Work out the finished part from the listing and answer in its coordinate system (mm). A direction names the side the tool comes from. Coordinates: 2 decimals unless noted, no trailing zeros. Order: outer loops, then holes, each group sorted by start corner. A loop starts at its lowest first (then second) coordinate and runs counter-clockwise, first axis right, second up. Notation, with made-up numbers: M 68.25,1.25 L 108.25,1.25 A7 cw 108.25,12.25 Z; hole C 51,-6.75 d9. An arc over 180 degrees is marked long. Write item = value, one per line. Start each with the question number.
Q1. Determine the mould class of faces 1 (the flat face through (-24.193, -41.132, 2.465)), 2 (the flat face through (24.193, 41.132, 2.465)), 3 (the cylindrical face through (41.745, 23.601, -0.253)) for opening direction Y: released by +Y, released by -Y, zero draft, split by the parting line, or undercut.
Q2. A tool of negligible diameter and unlimited length cuts with its end or side. For faces 4 (the flat face through (46, -19, 2)), 5 (the flat face through (-22.656, -38.519, 2.465)), 6 (the flat face through (-23.52, 41.52, 2.46)), from which of +Z, -Z, +X, -X, +Y, -Y can it reach the whole face along a straight path? Write none if from no direction.
Q3. Each of these flat-tipped pins is pushed along its axis until it touches: P1, Ø6.5, axis at x = 39.84, y = -23, coming from the +Z side; P2, Ø4, axis at y = 21, z = 3, coming from the -X side; P3, Ø4, axis at y = 12, z = 1.5, coming from the -X side; P4, Ø3.5, axis at x = 46.5, z = 2.5, coming from the -Y side. Where does it stop, or does it pass through?
Q4. Straight lines are drawn through the part: line 1 along Z through (x, y) = (13, -14.5); line 2 along X through (y, z) = (-47, -1.25); line 3 along X through (y, z) = (-46, -0.4). For each, find the intervals that lie inside material, in ascending order.
Q5. Find section C-C on y = 16.5. Give the vertices of the cut face in (x, z), and give its area (3 significant figures).
Q6. Find section B-B on z = 2.5. Give the vertices of the cut face in (x, y), and give its area (3 significant figures).
Q7. Find section A-A on y = -23. Give the vertices of the cut face in (x, z).
Q8. Find section D-D on x = -29.5. Give the vertices of the cut face in (y, z).
```python
from build123d import *

# Parameters (mm, degrees)
CYLINDER050_R            = 2
CYLINDER050_DEPTH        = 21
ARRAY002_COUNT           = 6
CYLINDER043_R            = 1.2
CYLINDER043_DEPTH        = 10
PRISM002_DEPTH           = 3
PRISM002_PLACEMENT_ANGLE = 30
BOX010_W                 = 5
BOX010_H                 = 38
BOX010_DEPTH             = 10
PRISM004_DEPTH           = 11
PRISM004_PLACEMENT_ANGLE = 30
PRISM003_DEPTH           = 5
PRISM003_PLACEMENT_ANGLE = 30
CHAMFER007_SIZE          = 2.5


with BuildPart() as agujeros_tornillos_tapa_inferior:
    # Cylinder050 → Cylinder050 (new body)
    with BuildSketch(Plane(origin=(0, -46, -8), x_dir=(1, 0, 0), z_dir=(0, 0, 1))):
        Circle(CYLINDER050_R)
    extrude(amount=CYLINDER050_DEPTH)

    # Array002: agujeros tornillos tapa inferior ×6 about axis
    array002_axis = Axis((0, 0, 0), (0, 0, 1))


with BuildPart() as agujeros_tornillos_tapa_inferior_1:
    add(agujeros_tornillos_tapa_inferior.part)
    for i in range(1, ARRAY002_COUNT):
        add(agujeros_tornillos_tapa_inferior.part.rotate(array002_axis, i * 360 / ARRAY002_COUNT))


with BuildPart() as cilindro019:
    # Cylinder043 → Cylinder043 (new body)
    with BuildSketch(Plane.XY.offset(-6)):
        Circle(CYLINDER043_R)
    extrude(amount=CYLINDER043_DEPTH)


with BuildPart() as obj1:
    # Prism002 → Prism002 (new body)
    with BuildSketch(Plane.XY):
        Polygon((58.5, 0), (29.25, 50.662486), (-29.25, 50.662486), (-58.5, 0), (-29.25, -50.662486), (29.25, -50.662486), align=None)
    extrude(amount=PRISM002_DEPTH)


with BuildPart() as obj1_1:
    # Prism002 placement: moved
    add(obj1.part.moved(Location((0, 0, -3))).rotate(Axis((0, 0, -3), (0, 0, 1)), PRISM002_PLACEMENT_ANGLE))

    # Cut011: cut Cilindro019
    add(cilindro019.part, mode=Mode.SUBTRACT)


with BuildPart() as cubo007:
    # Box010 → Box010 (new body)
    with BuildSketch(Plane(origin=(43.7, -19, 0), x_dir=(1, 0, 0), z_dir=(0, 0, 1))):
        with Locations((2.5, 19)):
            Rectangle(BOX010_W, BOX010_H)
    extrude(amount=BOX010_DEPTH)


with BuildPart() as tapa002:
    # Prism004 → Prism004 (new body)
    with BuildSketch(Plane.XY):
        Polygon((51.6, 0), (25.8, 44.686911), (-25.8, 44.686911), (-51.6, 0), (-25.8, -44.686911), (25.8, -44.686911), align=None)
    extrude(amount=PRISM004_DEPTH)


with BuildPart() as tapa002_1:
    # Prism004 placement: moved
    add(tapa002.part.rotate(Axis((0, 0, 0), (0, 0, 1)), PRISM004_PLACEMENT_ANGLE))


with BuildPart() as obj2:
    # Prism003 → Prism003 (new body)
    with BuildSketch(Plane.XY):
        Polygon((55.1, 0), (27.55, 47.718), (-27.55, 47.718), (-55.1, 0), (-27.55, -47.718), (27.55, -47.718), align=None)
    extrude(amount=PRISM003_DEPTH)


with BuildPart() as obj2_1:
    # Prism003 placement: moved
    add(obj2.part.rotate(Axis((0, 0, 0), (0, 0, 1)), PRISM003_PLACEMENT_ANGLE))

    # Cut006: cut tapa002
    add(tapa002_1.part, mode=Mode.SUBTRACT)

    # Cut007: cut Cubo007
    add(cubo007.part, mode=Mode.SUBTRACT)

    # Fusion006: union obj1
    add(obj1_1.part)

    # Cut021: cut agujeros tornillos tapa inferior
    add(agujeros_tornillos_tapa_inferior_1.part, mode=Mode.SUBTRACT)

    # Chamfer007
    chamfer007_edges = [obj2_1.edges().sort_by_distance(p)[0] for p in [
        (-2, -46, -3),
        (38.837169, -24.732051, -3),
        (2, 46, -3),
        (-38.837169, 24.732051, -3),
        (-40.837169, -21.267949, -3),
        (40.837169, 21.267949, -3),
    ]]
    chamfer(chamfer007_edges, length=CHAMFER007_SIZE)


solid = obj2_1.part
```
Findings below:
q1.face_1 = released by -Y
q1.face_2 = released by +Y
q1.face_3 = undercut
q2.face_4 = +Z, +X
q2.face_5 = +Z
q2.face_6 = +Z, -X, +Y
q3.P1 = 0
q3.P2 = -47.72
q3.P3 = -50.66
q3.P4 = -29.26
q4.line_1 = -3 to 0
q4.line_2 = -19.92 to -2.56, 2.56 to 19.92
q4.line_3 = -21.65 to -2, 2 to 21.65
q5.outline = M -50.66,-3 L 50.66,-3 L 50.66,0 L -44.69,0 L -44.69,5 L -47.72,5 L -47.72,0 L -50.66,0 Z
q5.area = 319 mm^2
q6.outline = M -47.72,-27.55 L 0,-55.1 L 47.72,-27.55 L 47.72,-19 L 44.69,-19 L 44.69,-25.8 L 0,-51.6 L -44.69,-25.8 L -44.69,25.8 L 0,51.6 L 44.69,25.8 L 44.69,19 L 47.72,19 L 47.72,27.55 L 0,55.1 L -47.72,27.55 Z
q6.area = 855 mm^2
q7.outline = M -50.66,-3 L -44.34,-3 L -41.84,-0.5 L -41.84,0 L -44.69,0 L -44.69,5 L -47.72,5 L -47.72,0 L -50.66,0 Z; M -37.84,-0.5 L -35.34,-3 L 35.34,-3 L 37.84,-0.5 L 37.84,0 L -37.84,0 Z; M 41.84,-0.5 L 44.34,-3 L 50.66,-3 L 50.66,0 L 47.72,0 L 47.72,5 L 44.69,5 L 44.69,0 L 41.84,0 Z
q8.outline = M -41.47,-3 L 41.47,-3 L 41.47,0 L 38.07,0 L 38.07,5 L 34.57,5 L 34.57,0 L -34.57,0 L -34.57,5 L -38.07,5 L -38.07,0 L -41.47,0 Z
